```python
from build123d import *

# Parameters (mm, degrees)
SKETCH1_W           = 23
SKETCH1_H           = 40
BOSS_EXTRUDE1_DEPTH = 20
SKETCH5_R           = 1.6
CUT_EXTRUDE3_DEPTH  = 21
SKETCH6_W           = 6
SKETCH6_H           = 2.5
CUT_EXTRUDE4_DEPTH  = 8
SKETCH7_R           = 2.8
CUT_EXTRUDE5_DEPTH  = 24
SKETCH8_R           = 5.5
CUT_EXTRUDE6_DEPTH  = 5
SKETCH9_W           = 13
SKETCH9_H           = 5.5
BOSS_EXTRUDE6_DEPTH = 2.5


with BuildPart() as part:
    # Sketch1 → Boss-Extrude1 (new body)
    with BuildSketch(Plane(origin=(0, 0, 0), x_dir=(1, 0, 0), z_dir=(0, 1, 0))):
        with Locations((10.80324178, 20)):
            Rectangle(SKETCH1_W, SKETCH1_H)
    extrude(amount=BOSS_EXTRUDE1_DEPTH)

    # Sketch5 → Cut-Extrude3 (cut, through all)
    with BuildSketch(Plane(origin=(0, 20, 0), x_dir=(1, 0, 0), z_dir=(0, 1, 0))):
        with Locations((18.30324178, 12)):
            Circle(SKETCH5_R)
        with Locations((18.30324178, 31)):
            Circle(SKETCH5_R)
    extrude(amount=-CUT_EXTRUDE3_DEPTH, mode=Mode.SUBTRACT)

    # Sketch6 → Cut-Extrude4 (cut)
    with BuildSketch(Plane(origin=(22.30324178, 0, 0), x_dir=(0, 0, -1), z_dir=(1, 0, 0))):
        with Locations((12, 15.75)):
            Rectangle(SKETCH6_W, SKETCH6_H)
        with Locations((31, 15.75)):
            Rectangle(SKETCH6_W, SKETCH6_H)
    extrude(amount=-CUT_EXTRUDE4_DEPTH, mode=Mode.SUBTRACT)

    # Sketch7 → Cut-Extrude5 (cut, through all)
    with BuildSketch(Plane.ZY.offset(0.69675822)):
        with Locations((-20, 10)):
            Circle(SKETCH7_R)
    extrude(amount=-CUT_EXTRUDE5_DEPTH, mode=Mode.SUBTRACT)

    # Sketch8 → Cut-Extrude6 (cut)
    with BuildSketch(Plane(origin=(22.30324178, 0, 0), x_dir=(0, 0, -1), z_dir=(1, 0, 0))):
        with Locations((20, 10)):
            Circle(SKETCH8_R)
    extrude(amount=-CUT_EXTRUDE6_DEPTH, mode=Mode.SUBTRACT)

    # Sketch9 → Boss-Extrude6 (add)
    with BuildSketch(Plane.ZY.offset(0.69675822)):
        with Locations((-33.5, 10)):
            Rectangle(SKETCH9_W, SKETCH9_H)
        with Locations((-6.5, 10)):
            Rectangle(SKETCH9_W, SKETCH9_H)
    extrude(amount=BOSS_EXTRUDE6_DEPTH)


solid = part.part
```
Model file for the job. Use its own axes, mm. A direction names the side the tool comes from. Coordinates: 2 decimals unless noted, no trailing zeros. Loops run counter-clockwise (first coordinate to the right, second up) from the corner with the lowest first, then second, coordinate; pieces in that order, holes last. Notation, with made-up numbers: (26, 47) - (44, 47) arc R28 ccw to (44, 83) - close; hole circle Ø9 at (5.5, -5). An arc over 180 degrees is marked (long way). Answer as a JSON object with one key per item and string values. Group by question number.
(1) Cut at C-C (x = 8.25). Give the cut face in (y, z), then the cut area to 3 significant figures.
(2) Cut at D-D (z = -20). Give the cut face in (x, y), then the cut area to 3 significant figures.
(3) Two-plate mould, pull along Y, no slides. Class faces 1 (the face through (-2, 7.25, -34)), 2 (the face through (20.1, 14.5, -12)), 3 (the face through (-2, 10, -27)): released by +Y, released by -Y, zero draft, split by the parting line, or undercut.
(4) Tool access for faces 4 (the face through (17.124, 7.352, -13.081)), 5 (the face through (-2, 12.75, -7)), 6 (the face through (-2, 7.25, -7)), 7 (the face through (18, 16, -9)): list every direction of +Z, -Z, +X, -X, +Y, -Y with a clear straight run to the whole face (end or side of a thin tool).
(5) Flat gauge pins, fed straight in: pin 1 (1.2 mm diameter, centred on y = 15.5, z = -31, fed in from +X); pin 2 (3.5 mm diameter, centred on y = 12, z = -18, fed in from +X); pin 3 (1.9 mm diameter, centred on x = 18.3, z = -12, fed in from -Y); pin 4 (9 mm diameter, centred on y = 10, z = -20, fed in from -X). Where does each tip first touch, or does it go through?
(6) Probe line 1 along Y through (x, z) = (11.75, -20); line 2 along X through (y, z) = (18.3, -31); line 3 along Y through (x, z) = (19.85, -20). List the from-to ranges inside material, lowest first.
(7) Cut at A-A (y = 10). Give the cut face in (x, z), then the cut area to 3 significant figures.
(8) Cut at B-B (z = -31). Give the cut face in (x, y).
Geometry says:
{
 "1": {"outline": "(0, -40) - (20, -40) - (20, 0) - (0, 0) - close; hole circle Ø5.6 at (10, -20)", "area": "775 mm^2"},
 "2": {"outline": "(-0.7, 0) - (22.3, 0) - (22.3, 4.5) - (17.3, 4.5) - (17.3, 7.2) - (-0.7, 7.2) - close; (-0.7, 12.8) - (17.3, 12.8) - (17.3, 15.5) - (22.3, 15.5) - (22.3, 20) - (-0.7, 20) - close", "area": "304 mm^2"},
 "3": {"face 1": "released by -Y", "face 2": "undercut", "face 3": "zero draft"},
 "4": {"face 4": "+Y, -Y", "face 5": "+Z, -Z, -X, +Y", "face 6": "+Z, -Z, -X, -Y", "face 7": "+X"},
 "5": {"pin 1": "stops at x = 14.3", "pin 2": "stops at x = 17.3", "pin 3": "passes through", "pin 4": "stops at x = -0.7"},
 "6": {"line 1": "y = 0 to 7.2, 12.8 to 20", "line 2": "x = -0.7 to 16.7, 19.9 to 22.3", "line 3": "y = 0 to 4.5, 15.5 to 20"},
 "7": {"outline": "(-3.2, -40) - (22.3, -40) - (22.3, -25.5) - (17.3, -25.5) - (17.3, -22.8) - (-0.7, -22.8) - (-0.7, -27) - (-3.2, -27) - close; (-3.2, -13) - (-0.7, -13) - (-0.7, -17.2) - (17.3, -17.2) - (17.3, -14.5) - (22.3, -14.5) - (22.3, 0) - (-3.2, 0) - close; hole circle Ø3.2 at (18.3, -31); hole circle Ø3.2 at (18.3, -12)", "area": "813 mm^2"},
 "8": {"outline": "(-3.2, 7.25) - (-0.7, 7.25) - (-0.7, 0) - (16.7, 0) - (16.7, 14.5) - (14.3, 14.5) - (14.3, 17) - (16.7, 17) - (16.7, 20) - (-0.7, 20) - (-0.7, 12.75) - (-3.2, 12.75) - close; (19.9, 0) - (22.3, 0) - (22.3, 14.5) - (19.9, 14.5) - close; (19.9, 17) - (22.3, 17) - (22.3, 20) - (19.9, 20) - close"}
}
